Check sheet for the modelled part. Datum: model origin and axes. Units: mm. Face numbers are marked on the shaded views. A direction names the side the tool comes from. Coordinates: 2 decimals unless noted, no trailing zeros. Write each loop counter-clockwise with the first axis right and the second up, starting at its lowest first coordinate (ties: lowest second). Pieces come first, ordered by that corner, then holes. Notation, with made-up numbers: (18.25, 42.5) - (72.25, 42.5) arc R26 ccw to (72.25, 65.5) - close; hole circle Ø2 at (23, 67). An arc over 180 degrees is marked (long way). Use one line per item in the form item = value. Start each with the question number.
1. Cross-section at A-A on y = -1.5. Record the boundary of the cut face in (x, z).
2. Draft check along Y on the marked faces 1, 2 and 3. Enter one of: +Y half, -Y half, draft (parallel to the pull), parting line (faces both ways), or undercut.
3. Cross-section at C-C on y = -23. Record the boundary of the cut face in (x, z), then the cut area to 3 significant figures.
4. Go/stop test with flat-tipped pins: pin 1 Ø0.9 at (y, z) = (-19.5, 2) entering from +X; pin 2 Ø8 at (x, y) = (-5, 4) entering from -Z; pin 3 Ø1.5 at (y, z) = (4, 2.5) entering from -X. Record where each tip stops, or that it passes through.
5. Tool access check on the marked faces 4, 5, 6, 7 and 8. Record the directions out of +Z, -Z, +X, -X, +Y, -Y that give a thin tool (end or side, any length) a straight path to the whole face; none if there is none.
6. Scan lines: line 1 along Y through (x, z) = (15, 2); line 2 along Y through (x, z) = (-5.5, 1.35); line 3 along Y through (x, z) = (-10.5, 1.8). Record each from-to range of solid material in increasing order.
7. Cross-section at B-B on z = 1.7. Record the boundary of the cut face in (x, y).
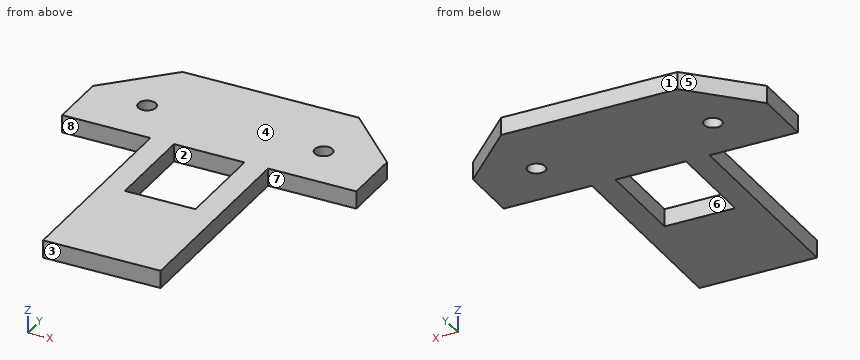
```python
from build123d import *

# Parameters (mm, degrees)
CROQUIS1_R              = 1.5
CROQUIS1_W              = 12
CROQUIS1_H              = 16
SALIENTE_EXTRUIR1_DEPTH = 3


with BuildPart() as part:
    # Croquis1 → Saliente-Extruir1 (new body)
    with BuildSketch(Plane.XY):
        Polygon((-25, 0), (-15, 10), (15, 10), (25, 0), (25, -10), (10, -10), (10, -45), (-10, -45), (-10, -10), (-25, -10), align=None)
        with Locations((-15, -1.5)):
            Circle(CROQUIS1_R, mode=Mode.SUBTRACT)
        with Locations((15, -1.5)):
            Circle(CROQUIS1_R, mode=Mode.SUBTRACT)
        with Locations((0, -18)):
            Rectangle(CROQUIS1_W, CROQUIS1_H, mode=Mode.SUBTRACT)
    extrude(amount=SALIENTE_EXTRUIR1_DEPTH)


solid = part.part
```
Final values:
q1.outline = (-25, 0) - (-16.5, 0) - (-16.5, 3) - (-25, 3) - close; (-13.5, 0) - (13.5, 0) - (13.5, 3) - (-13.5, 3) - close; (16.5, 0) - (25, 0) - (25, 3) - (16.5, 3) - close
q2.face_1 = +Y half
q2.face_2 = undercut
q2.face_3 = -Y half
q3.outline = (-10, 0) - (-6, 0) - (-6, 3) - (-10, 3) - close; (6, 0) - (10, 0) - (10, 3) - (6, 3) - close
q3.area = 24.0 mm²
q4.pin_1 = 10
q4.pin_2 = 0
q4.pin_3 = -21.75
q5.face_4 = +Z, +X, -X, +Y, -Y
q5.face_5 = +Z, -Z, -X, +Y
q5.face_6 = +Z, -Z
q5.face_7 = +Z, -Z, +X, -Y
q5.face_8 = +Z, -Z, -X, -Y
q6.line_1 = -10 to -3, 0 to 10
q6.line_2 = -45 to -26, -10 to 10
q6.line_3 = -10 to 10
q7.outline = (-25, -10) - (-10, -10) - (-10, -45) - (10, -45) - (10, -10) - (25, -10) - (25, 0) - (15, 10) - (-15, 10) - (-25, 0) - close; hole circle Ø3 at (-15, -1.5); hole (-6, -26) - (6, -26) - (6, -10) - (-6, -10) - close; hole circle Ø3 at (15, -1.5)
